Read the model definition and answer for the solid it produces. Units are mm, in the model's axes. Coordinates: 2 decimals unless noted, no trailing zeros. Write each loop counter-clockwise with the first axis right and the second up, starting at its lowest first coordinate (ties: lowest second). Pieces come first, ordered by that corner, then holes. Notation, with made-up numbers: (-31.5, 51.25) -> (25.5, 51.25) arc R20 cw to (25.5, 88.25) -> close; hole circle Ø1 at (41.5, 76). An arc over 180 degrees is marked (long way). Return JSON: item names as keys, results as strings.
from build123d import *

# Parameters (mm, degrees)
F0_W     = 57.15
F0_H     = 38.1
F1_DEPTH = 25.4
F3_DEPTH = 25.4
F5_DEPTH = 25.4


with BuildPart() as f1:
    # F0 (on Front) → F1 (new body)
    with BuildSketch(Plane.XZ):
        with Locations((28.575, 19.05)):
            Rectangle(F0_W, F0_H)
    extrude(amount=-F1_DEPTH)

    # F2 (on Front) → F3 (cut)
    with BuildSketch(Plane.XZ):
        with BuildLine():
            Line((57.15, 38.1), (38.1, 38.1))
            ThreePointArc((38.1, 38.1), (43.679616, 24.629616), (57.15, 19.05))
            Line((57.15, 19.05), (57.15, 38.1))
        make_face()
    extrude(amount=-F3_DEPTH, mode=Mode.SUBTRACT)

    # F4 (on Front) → F5 (cut)
    with BuildSketch(Plane.XZ):
        with BuildLine():
            ThreePointArc((0, 25.4), (3.719744, 34.380256), (12.7, 38.1))
            Line((12.7, 38.1), (0, 38.1))
            Line((0, 38.1), (0, 25.4))
        make_face()
    extrude(amount=-F5_DEPTH, mode=Mode.SUBTRACT)


solid = f1.part
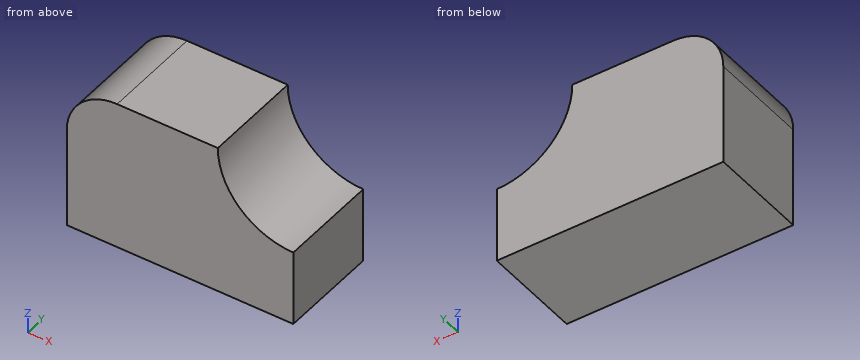
1. Flat-ended cylindrical pins translate along their axes: pin 1 Ø4 at (y, z) = (11, 27) entering from +X; pin 2 Ø1 at (x, y) = (48, 9.5) entering from +Z (3 decimals). Find the tip coordinate at first contact, or state that the pin passes through.
Taken from the geometry:
{"pin 1": "stops at x = 43.32", "pin 2": "stops at z = 21.675"}
2. The part is cut by section A-A (y = 13.25). Determine the outline of the cut face in (x, z).
Taken from the geometry:
{"outline": "(0, 0) -> (57.15, 0) -> (57.15, 19.05) arc R19.05 cw to (38.1, 38.1) -> (12.7, 38.1) arc R12.7 ccw to (0, 25.4) -> close"}
3. The part is cut by section C-C (x = 39.5). Determine the outline of the cut face in (y, z).
Taken from the geometry:
{"outline": "(0, 0) -> (25.4, 0) -> (25.4, 30.93) -> (0, 30.93) -> close"}
4. Consider L1, parallel to X at y = 14.75, z = 35; L2, parallel to Z at x = 5.5, y = 2.25; L3, parallel to X at y = 17.5, z = 27.5. Determine where each line is inside the solid, lowest interval first.
Taken from the geometry:
{"L1": "x = 4.39 to 38.35", "L2": "z = 0 to 35.86", "L3": "x = 0.17 to 41.32"}
5. The part is cut by section B-B (z = 32). Determine the outline of the cut face in (x, y).
Taken from the geometry:
{"outline": "(1.85, 0) -> (39.1, 0) -> (39.1, 25.4) -> (1.85, 25.4) -> close"}
